Input: part model. Units: mm. Frame: model coordinates. A direction names the side the tool comes from. Round coordinates to 2 decimals unless told otherwise and drop trailing zeros. Loops run counter-clockwise (first coordinate to the right, second up) from the corner with the lowest first, then second, coordinate; pieces in that order, holes last. Notation, with made-up numbers: M 21,-39.75 L 28,-39.75 A11 cw 28,-33.75 Z; hole C -7.5,61.25 d4. An arc over 180 degrees is marked long. Put each result on its own line as item: value. Start each with the question number.
1) Draft query along Z for faces 1 (the face through (-15, 13, 10)), 2 (the face through (-5, 13, -10)), 3 (the face through (-5, 13, 60)), 4 (the face through (-2.69, 5.07, 64.96)). Return one class per face: +Z half, -Z half, draft (parallel to the pull), parting line (faces both ways), or undercut.
2) Section B-B on x = -5. Output: boundary loops of the cut face in (y, z), plus the area to 3 significant figures.
3) Section D-D on y = 7.75. Output: boundary loops of the cut face in (x, z).
4) Line query: probe 1 along Z at (x, y) = (15, 7.5); probe 2 along Z at (x, y) = (-29, 6); probe 3 along X at (y, z) = (11, -3.5). Output: solid intervals per line, ascending.
5) Reachability of faces 5 (the face through (-15, 5, 45)), 6 (the face through (-20, 13, -7.2)), 7 (the face through (-20, 13, -12.8)), 8 (the face through (-15, 13, -10)) from +Z, -Z, +X, -X, +Y, -Y: full face, straight path, thin tool, end or side. Return the list, or none.
6) Pin query (flat end, axial travel): pin 1 (12 mm diameter, centred on x = -8.5, z = 60.5, fed in from +Y); pin 2 (2 mm diameter, centred on x = 6, z = 26, fed in from +Y); pin 3 (3 mm diameter, centred on y = 13, z = 9, fed in from +X); pin 4 (1.7 mm diameter, centred on x = -4, y = 12, fed in from -Z). Return the tip coordinate at first contact, or that it passes through.
7) Section C-C on z = 10. Output: boundary loops of the cut face in (x, y).
8) Section A-A on y = 14. Output: boundary loops of the cut face in (x, z).
from build123d import *

# Parameters (mm, degrees)
SALIENTE_EXTRUIR1_DEPTH = 10
SALIENTE_EXTRUIR2_DEPTH = 90
SALIENTE_EXTRUIR3_DEPTH = 50
CROQUIS6_W              = 56.928573576
CROQUIS6_H              = 55.923287038
CORTAR_EXTRUIR2_DEPTH   = 30
CROQUIS5_W              = 40
CROQUIS5_H              = 10
CROQUIS5_W_2            = 10
CROQUIS5_H_2            = 40
CORTAR_EXTRUIR1_DEPTH   = 5.7
CROQUIS7_R              = 2.5
CORTAR_EXTRUIR3_DEPTH   = 11


with BuildPart() as part:
    # Croquis1 → Saliente-Extruir1 (new body)
    with BuildSketch(Plane(origin=(0, 0, 0), x_dir=(1, 0, 0), z_dir=(0, 1, 0))):
        Polygon((25, 20), (-65, 20), (-65, -20), (-15, -20), (-15, -70), (25, -70), (25, -20), align=None)
    extrude(amount=SALIENTE_EXTRUIR1_DEPTH)

    # Croquis2 → Saliente-Extruir2 (add, through all)
    with BuildSketch(Plane.XY.offset(70)):
        Polygon((12.2, 9.987376579), (12.2, 15.7), (17.8, 15.7), (17.8, 9.987376579), (15, 9.987376579), align=None)
        Polygon((-7.8, 9.987376579), (-7.8, 15.7), (-2.2, 15.7), (-2.2, 9.987376579), (-5, 9.987376579), align=None)
    extrude(amount=-SALIENTE_EXTRUIR2_DEPTH)

    # Croquis3 → Saliente-Extruir3 (add)
    with BuildSketch(Plane.ZY.offset(65)):
        Polygon((7.2, 10), (7.2, 15.7), (12.8, 15.7), (12.8, 10), (10, 10), align=None)
        Polygon((-12.8, 10), (-12.8, 15.7), (-7.2, 15.7), (-7.2, 10), (-10, 10), align=None)
    extrude(amount=-SALIENTE_EXTRUIR3_DEPTH)

    # Croquis6 → Cortar-Extruir2 (cut)
    with BuildSketch(Plane.ZY.offset(65)):
        Rectangle(CROQUIS6_W, CROQUIS6_H)
    extrude(amount=-CORTAR_EXTRUIR2_DEPTH, mode=Mode.SUBTRACT)

    # Croquis5 → Cortar-Extruir1 (cut)
    with BuildSketch(Plane(origin=(0, 15.7, 0), x_dir=(1, 0, 0), z_dir=(0, 1, 0))):
        with Locations((5, -65)):
            Rectangle(CROQUIS5_W, CROQUIS5_H)
        with Locations((5, 15)):
            Rectangle(CROQUIS5_W, CROQUIS5_H)
        with Locations((-30, 0)):
            Rectangle(CROQUIS5_W_2, CROQUIS5_H_2)
    extrude(amount=-CORTAR_EXTRUIR1_DEPTH, mode=Mode.SUBTRACT)

    # Croquis7 → Cortar-Extruir3 (cut, through all)
    with BuildSketch(Plane(origin=(0, 10, 0), x_dir=(1, 0, 0), z_dir=(0, 1, 0))):
        with Locations((-29, 10)):
            Circle(CROQUIS7_R)
        with Locations((-29, -10)):
            Circle(CROQUIS7_R)
        with Locations((15, 14)):
            Circle(CROQUIS7_R)
        with Locations((-5, 14)):
            Circle(CROQUIS7_R)
        with Locations((-5, -64)):
            Circle(CROQUIS7_R)
        with Locations((15, -64)):
            Circle(CROQUIS7_R)
    extrude(amount=-CORTAR_EXTRUIR3_DEPTH, mode=Mode.SUBTRACT)


solid = part.part
Geometry results:
1. face 1: draft
1. face 2: -Z half
1. face 3: +Z half
1. face 4: undercut
2. outline: M 0,-20 L 10,-20 L 10,-16.5 L 0,-16.5 Z; M 0,-11.5 L 10,-11.5 L 10,-10 L 15.7,-10 L 15.7,60 L 10,60 L 10,61.5 L 0,61.5 Z; M 0,66.5 L 10,66.5 L 10,70 L 0,70 Z
2. area: 1,200 mm²
3. outline: M -35,-20 L 25,-20 L 25,70 L -15,70 L -15,20 L -35,20 Z; hole C -29,-10 d5; hole C -29,10 d5; hole C -5,-14 d5; hole C -5,64 d5; hole C 15,-14 d5; hole C 15,64 d5
4. probe 1: z = -20 to -16.5, -11.5 to 61.5, 66.5 to 70
4. probe 2: z = -20 to -12.5, -7.5 to 7.5, 12.5 to 20
4. probe 3: x = -7.8 to -2.2, 12.2 to 17.8
5. face 5: +Z, -X, +Y, -Y
5. face 6: -X, +Y
5. face 7: -Z, +X, -X, +Y
5. face 8: +Z, -Z, +Y
6. pin 1: stops at y = 15.7
6. pin 2: stops at y = 10
6. pin 3: stops at x = 17.8
6. pin 4: stops at z = -10
7. outline: M -35,0 L -31.5,0 L -31.5,10 L -35,10 Z; M -26.5,0 L 25,0 L 25,10 L 17.8,10 L 17.8,15.7 L 12.2,15.7 L 12.2,10 L -2.2,10 L -2.2,15.7 L -7.8,15.7 L -7.8,10 L -15,10 L -15,15.7 L -25,15.7 L -25,10 L -26.5,10 Z
8. outline: M -25,-12.8 L -15,-12.8 L -15,-7.2 L -25,-7.2 Z; M -25,7.2 L -15,7.2 L -15,12.8 L -25,12.8 Z; M -7.8,-10 L -2.2,-10 L -2.2,60 L -7.8,60 Z; M 12.2,-10 L 17.8,-10 L 17.8,60 L 12.2,60 Z
